Here's the drawing with two shaded views (mm, measured from the low corner). I have some questions. Give positions to 0.01 mm unless a question says otherwise; leave off trailing zeros. Loops run counter-clockwise (first coordinate to the right, second up) from the corner with the lowest first, then second, coordinate; pieces in that order, holes last. Notation, with made-up numbers: (36.5, -8) - (61.5, -8) arc R5 cw to (61.5, -2) - close; hole circle Ø4 at (71, -21.5). An arc over 180 degrees is marked (long way). Write each question's results on one line, items separated by ' | '. Start each with the question number.
1) I want a section at C-C, the plane x = 40.5. Write out the boundary of the cut face in (y, z), and give its area (3 significant figures).
2) I want a section at D-D, the plane y = 63. Write out the boundary of the cut face in (x, z).
3) I want a section at A-A, the plane y = 20. Write out the boundary of the cut face in (x, z), and give its area (4 significant figures).
4) If I drill on probe 1 along Y at (x, z) = (40.5, 1.55); probe 2 along X at (y, z) = (61.5, 2.25); probe 3 along X at (y, z) = (65.5, 2.8), over which ranges is the centre line in solid material (lowest first)? Write a range as [from, to].
5) I want a section at B-B, the plane z = 0.9. Write out the boundary of the cut face in (x, y), and give its area (3 significant figures).
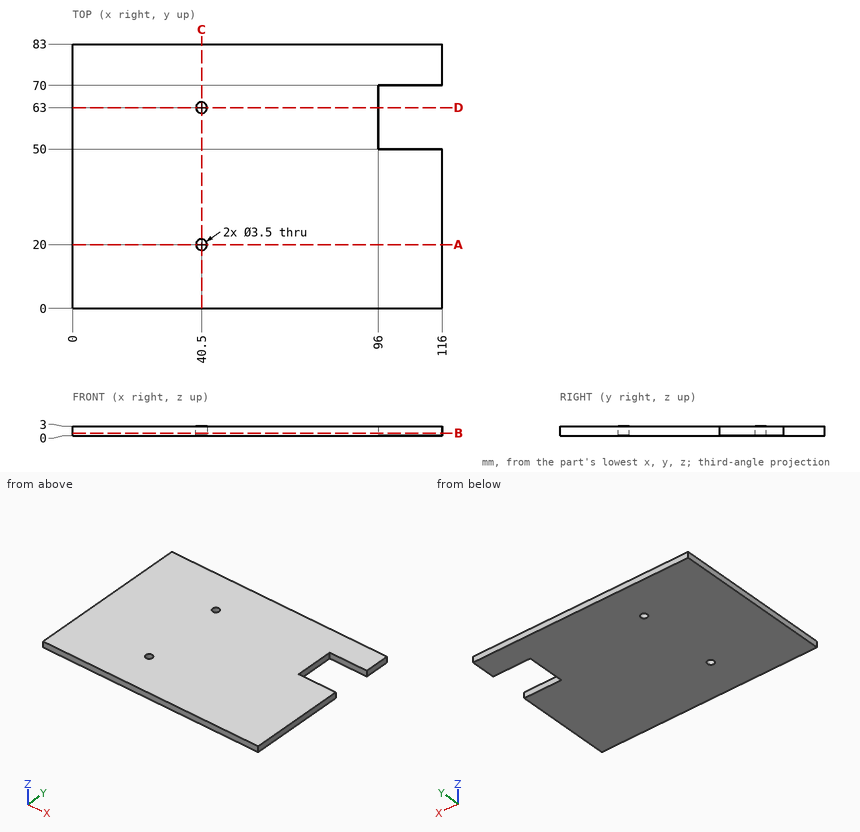
Answers:
1) outline: (0, 0) - (18.25, 0) - (18.25, 3) - (0, 3) - close; (21.75, 0) - (61.25, 0) - (61.25, 3) - (21.75, 3) - close; (64.75, 0) - (83, 0) - (83, 3) - (64.75, 3) - close | area: 228 mm2
2) outline: (0, 0) - (38.75, 0) - (38.75, 3) - (0, 3) - close; (42.25, 0) - (96, 0) - (96, 3) - (42.25, 3) - close
3) outline: (0, 0) - (38.75, 0) - (38.75, 3) - (0, 3) - close; (42.25, 0) - (116, 0) - (116, 3) - (42.25, 3) - close | area: 337.5 mm2
4) probe 1: y = [0, 18.25], [21.75, 61.25], [64.75, 83] | probe 2: x = [0, 39.6], [41.4, 96] | probe 3: x = [0, 96]
5) outline: (0, 0) - (116, 0) - (116, 50) - (96, 50) - (96, 70) - (116, 70) - (116, 83) - (0, 83) - close; hole circle Ø3.5 at (40.5, 20); hole circle Ø3.5 at (40.5, 63) | area: 9,210 mm2
